```python
from build123d import *

# Parameters (mm, degrees)
SKETCH1_R               = 2.38125
BOSS_EXTRUDE1_DEPTH     = 6.35
CUT_EXTRUDE1_DEPTH      = 42.152703435
CUT_EXTRUDE1_DEPTH_BACK = 42.152703435
SKETCH2_R               = 2.38125
FILLET1_R               = 6.35
FILLET2_R               = 4.7625
CHAMFER1_SIZE           = 0.396875


with BuildPart() as part:
    # Sketch1 → Boss-Extrude1 (new, symmetric)
    with BuildSketch(Plane(origin=(0, 0, 0), x_dir=(1, 0, 0), z_dir=(0, 1, 0))):
        Polygon((-6.35, -6.35), (31.75, -6.35), (31.75, 0), (4.7625, 0), (4.7625, 19.05), (-6.35, 19.05), align=None)
        with Locations(Location((0, 0, 0), (0, 0, 270))):
            Circle(SKETCH1_R, mode=Mode.SUBTRACT)
        with Locations(Location((0, 12.7, 0), (0, 0, 270))):
            Circle(SKETCH1_R, mode=Mode.SUBTRACT)
    extrude(amount=BOSS_EXTRUDE1_DEPTH, both=True)

    # Sketch2 → Cut-Extrude1 (cut, two sides: drawn at the far end of the back side and taken through both)
    with BuildSketch(Plane.XY.offset(6.35).offset(-CUT_EXTRUDE1_DEPTH_BACK)):
        with Locations((25.4, 0)):
            Circle(SKETCH2_R)
    extrude(amount=CUT_EXTRUDE1_DEPTH + CUT_EXTRUDE1_DEPTH_BACK, mode=Mode.SUBTRACT)

    # Fillet1
    fillet1_edges = [part.edges().sort_by_distance(p)[0] for p in [
        (-6.35, 0, -19.05),
        (4.7625, 0, 0),
        (31.75, -6.35, 3.175),
        (31.75, 6.35, 3.175),
    ]]
    fillet(fillet1_edges, radius=FILLET1_R - 0.0001)  # a hair under: the kernel refuses the full size

    # Fillet2
    fillet2_edges = [part.edges().sort_by_distance(p)[0] for p in [
        (-6.35, 0, 6.35),
        (4.7625, 0, -19.05),
    ]]
    fillet(fillet2_edges, radius=FILLET2_R)

    # Chamfer1
    chamfer1_edges = [part.edges().sort_by_distance(p)[0] for p in [
        (0, -6.35, -2.38125),
        (0, 6.35, -2.38125),
        (0, -6.35, -15.08125),
        (0, 6.35, -15.08125),
        (23.01875, 0, 0),
        (23.01875, 0, 6.35),
        (-6.35, -6.35, -5.5563),
        (-6.35, 6.35, -5.5563),
        (4.7625, -6.35, -10.3187),
        (18.25625, -6.35, 0),
        (-4.49015735, -6.35, -17.19015735),
        (18.25625, 6.35, 0),
        (4.7625, 6.35, -10.3187),
        (-4.49015735, 6.35, -17.19015735),
        (29.89015735, 4.49015735, 0),
        (29.89015735, -4.49015735, 0),
        (29.89015735, 4.49015735, 6.35),
        (29.89015735, -4.49015735, 6.35),
        (6.62234265, -6.35, -1.85984265),
        (6.62234265, 6.35, -1.85984265),
        (11.9063, -6.35, 6.35),
        (11.9063, 6.35, 6.35),
        (3.367596045, -6.35, -17.655096045),
        (-4.955096045, -6.35, 4.955096045),
        (3.367596045, 6.35, -17.655096045),
        (-4.955096045, 6.35, 4.955096045),
    ]]
    chamfer(chamfer1_edges, length=CHAMFER1_SIZE)


solid = part.part
```
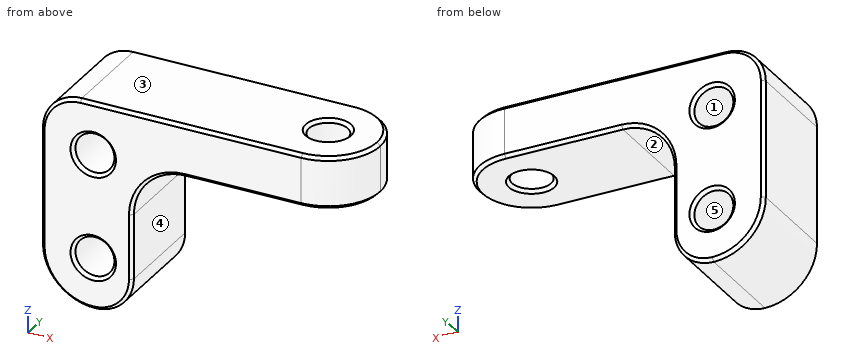
Geometry check sheet. Reference: the model listing, model coordinates, mm. Face numbers are marked on the shaded views. A direction names the side the tool comes from. Round coordinates to 2 decimals unless told otherwise and drop trailing zeros. Order: outer loops, then holes, each group sorted by start corner. A loop starts at its lowest first (then second) coordinate and runs counter-clockwise, first axis right, second up. Notation, with made-up numbers: M -4.75,15.5 L 16.25,15.5 A15 cw 16.25,21.5 Z; hole C 21,37.5 d4. An arc over 180 degrees is marked long. Answer as CSV lines item,"result".
1) Thickness scan on probe 1 along X at (y, z) = (5, -12.75); probe 2 along Y at (x, z) = (25.4, 1.85). Record the ranges inside material, lowest first. Write a range as [from, to].
Entries:
probe 1,"[-6.35, -2.38], [2.38, 4.76]"
probe 2,"[-6.35, -2.38], [2.38, 6.35]"
2) Gauge pin test, flat ends, axial feed: pin 1 Ø2.5 at (y, z) = (0, -9) entering from +X; pin 2 Ø5 at (x, z) = (0, 0) entering from +Y; pin 3 Ø5 at (x, y) = (23, 0.5) entering from -Z; pin 4 Ø4 at (x, z) = (24.5, -2.5) entering from +Y. Record the tip position at first contact, or that the pin passes through.
Entries:
pin 1,"x = 4.76"
pin 2,"y = 6.07"
pin 3,"z = 0"
pin 4,"through"
3) Sectioned sample at C-C on y = 0.75. Give the number of separate pieces and of enclosed holes in the cut face, and give its area (3 significant figures).
Entries:
separate pieces,"2"
enclosed holes,"2"
area,"379 mm2"
4) Sectioned sample at A-A on z = -8. Record the cut outline in (x, y), and give its area (3 significant figures).
Entries:
outline,"M -6.35,-5.95 L -5.95,-6.35 L 4.37,-6.35 L 4.76,-5.95 L 4.76,5.95 L 4.37,6.35 L -5.95,6.35 L -6.35,5.95 Z"
area,"141 mm2"
5) Mould release check, pull along Z, two halves, no side actions. Record for the marked faces 1, 2 and 3: +Z half, -Z half, draft (parallel to the pull), parting line (faces both ways), or undercut.
Entries:
face 1,"undercut"
face 2,"-Z half"
face 3,"+Z half"
6) Tool access check on the marked faces 4 and 5. Record the directions out of +Z, -Z, +X, -X, +Y, -Y that give a thin tool (end or side, any length) a straight path to the whole face; none if there is none.
Entries:
face 4,"-Z, +X, +Y, -Y"
face 5,"+Y, -Y"
7) Sectioned sample at B-B on x = 21.5. Record the cut outline in (y, z).
Entries:
outline,"M -6.35,0.4 L -5.95,0 L 5.95,0 L 6.35,0.4 L 6.35,5.95 L 5.95,6.35 L -5.95,6.35 L -6.35,5.95 Z"
